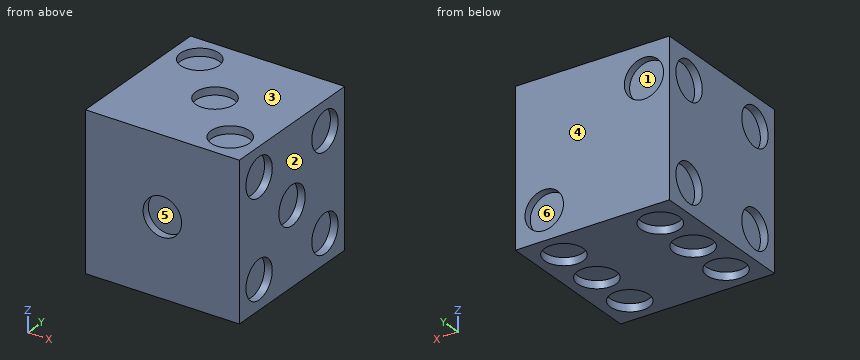
from build123d import *

# Parameters (mm, degrees)
F0_W      = 8
F0_H      = 8
F1_DEPTH  = 8
F2_R      = 1
F3_DEPTH  = 0.4
F4_R      = 1
F4_R_2    = 1.018966
F5_DEPTH  = 0.4
F6_R      = 1
F7_DEPTH  = 0.4
F8_R      = 1
F9_DEPTH  = 0.4
F10_R     = 1
F11_DEPTH = 0.4
F12_R     = 1
F13_DEPTH = 0.4


with BuildPart() as f1:
    # F0 (on Front) → F1 (new body)
    with BuildSketch(Plane.XZ):
        with Locations((2.040328, 4.226393)):
            Rectangle(F0_W, F0_H)
    extrude(amount=F1_DEPTH)

    # F2 (on face) → F3 (cut)
    with BuildSketch(Plane.XZ.offset(8)):
        with Locations((2.040328, 4.226393)):
            Circle(F2_R)
    extrude(amount=-F3_DEPTH, mode=Mode.SUBTRACT)

    # F4 (on face) → F5 (cut)
    with BuildSketch(Plane(origin=(0, 0, 0), x_dir=(-1, 0, 0), z_dir=(0, 1, 0))):
        with Locations((-4.540328, 1.726393)):
            Circle(F4_R)
        with Locations((0.640184, 6.564468)):
            Circle(F4_R_2)
    extrude(amount=-F5_DEPTH, mode=Mode.SUBTRACT)

    # F6 (on face) → F7 (cut)
    with BuildSketch(Plane(origin=(-1.959672, 0, 0), x_dir=(0, -1, 0), z_dir=(-1, 0, 0))):
        with Locations((6.5, 6.726393)):
            Circle(F6_R)
        with Locations((1.5, 6.726393)):
            Circle(F6_R)
        with Locations((1.5, 1.726393)):
            Circle(F6_R)
        with Locations((6.5, 1.726393)):
            Circle(F6_R)
    extrude(amount=-F7_DEPTH, mode=Mode.SUBTRACT)

    # F8 (on face) → F9 (cut)
    with BuildSketch(Plane.YZ.offset(6.040328)):
        with Locations((-4, 4.226393)):
            Circle(F8_R)
        with Locations((-6.5, 6.726393)):
            Circle(F8_R)
        with Locations((-1.5, 6.726393)):
            Circle(F8_R)
        with Locations((-1.5, 1.726393)):
            Circle(F8_R)
        with Locations((-6.5, 1.726393)):
            Circle(F8_R)
    extrude(amount=-F9_DEPTH, mode=Mode.SUBTRACT)

    # F10 (on face) → F11 (cut)
    with BuildSketch(Plane.XY.offset(8.226393)):
        with Locations((-0.459672, -1.5)):
            Circle(F10_R)
        with Locations((2.040328, -4)):
            Circle(F10_R)
        with Locations((4.540328, -6.5)):
            Circle(F10_R)
    extrude(amount=-F11_DEPTH, mode=Mode.SUBTRACT)

    # F12 (on face) → F13 (cut)
    with BuildSketch(Plane(origin=(0, 0, 0.226393), x_dir=(1, 0, 0), z_dir=(0, 0, -1))):
        with Locations((-0.459672, 6.5)):
            Circle(F12_R)
        with Locations((-0.459672, 4)):
            Circle(F12_R)
        with Locations((-0.459672, 1.5)):
            Circle(F12_R)
        with Locations((4.540328, 1.5)):
            Circle(F12_R)
        with Locations((4.540328, 4)):
            Circle(F12_R)
        with Locations((4.540328, 6.5)):
            Circle(F12_R)
    extrude(amount=-F13_DEPTH, mode=Mode.SUBTRACT)


solid = f1.part
Here's how the part is built. I have some questions about the finished solid (model axes, mm). Face numbers are marked on the shaded views. A direction names the side the tool comes from. Give positions to 0.01 mm unless a question says otherwise; leave off trailing zeros. Order: outer loops, then holes, each group sorted by start corner. A loop starts at its lowest first (then second) coordinate and runs counter-clockwise, first axis right, second up. Notation, with made-up numbers: (80, 85.25) -> (118, 85.25) arc R18 cw to (118, 98.25) -> close; hole circle Ø1 at (22, -36). An arc over 180 degrees is marked (long way). One line per item, written item: value. Start each with the question number.
1. Will these pins go through, and if not, where does the flat tip stop? pin 1 Ø1 at (y, z) = (-7, 6) entering from -X; pin 2 Ø1.6 at (y, z) = (-6.5, 6.73) entering from +X; pin 3 Ø0.6 at (x, z) = (2.5, 4) entering from -Y; pin 4 Ø0.6 at (x, y) = (4, -4) entering from -Z.
2. Imagine slicing it at B-B, the plane z = 1. List the corners of the cut face in (x, y) for me, plus the area to 3 significant figures.
3. Imagine slicing it at A-A, the plane y = -4. List the corners of the cut face in (x, z) for me.
4. For the marked faces 4, 5 and 6, which set-ups out of +Z, -Z, +X, -X, +Y, -Y let a thin tool reach every point of the face, with its end or its side?
5. I need wall thicknesses on probe 1 along X at (y, z) = (-1.5, 0.35); probe 2 along Z at (x, y) = (5.9, -6.5); probe 3 along Z at (x, y) = (4.25, -3.5). Which ranges of each line are inside material? Lowest first, please. Write a range as from..to.
6. Imagine slicing it at C-C, the plane x = 2. List the corners of the cut face in (y, z) for me, plus the area to 3 significant figures.
7. We'd pull the mould along X, two halves only. Please class the marked faces 1, 2 and 3: released by +X, released by -X, zero draft, split by the parting line, or undercut.
Values follow:
1. pin 1: stops at x = -1.96
1. pin 2: stops at x = 5.64
1. pin 3: stops at y = -7.6
1. pin 4: stops at z = 0.63
2. outline: (-1.96, -8) -> (6.04, -8) -> (6.04, -7.19) -> (5.64, -7.19) -> (5.64, -5.81) -> (6.04, -5.81) -> (6.04, -2.19) -> (5.64, -2.19) -> (5.64, -0.81) -> (6.04, -0.81) -> (6.04, 0) -> (5.23, 0) -> (5.23, -0.4) -> (3.85, -0.4) -> (3.85, 0) -> (-1.96, 0) -> (-1.96, -0.81) -> (-1.56, -0.81) -> (-1.56, -2.19) -> (-1.96, -2.19) -> (-1.96, -5.81) -> (-1.56, -5.81) -> (-1.56, -7.19) -> (-1.96, -7.19) -> close
2. area: 61.3 mm2
3. outline: (-1.96, 0.23) -> (-1.46, 0.23) -> (-1.46, 0.63) -> (0.54, 0.63) -> (0.54, 0.23) -> (3.54, 0.23) -> (3.54, 0.63) -> (5.54, 0.63) -> (5.54, 0.23) -> (6.04, 0.23) -> (6.04, 3.23) -> (5.64, 3.23) -> (5.64, 5.23) -> (6.04, 5.23) -> (6.04, 8.23) -> (3.04, 8.23) -> (3.04, 7.83) -> (1.04, 7.83) -> (1.04, 8.23) -> (-1.96, 8.23) -> close
4. face 4: +Z, -Z, +X, -X, +Y
4. face 5: -Y
4. face 6: +Y
5. probe 1: x = -1.96..-1.46, 0.54..3.54, 5.54..6.04
5. probe 2: z = 0.23..0.73, 2.73..5.73, 7.73..8.23
5. probe 3: z = 0.63..8.23
6. outline: (-8, 0.23) -> (0, 0.23) -> (0, 8.23) -> (-3, 8.23) -> (-3, 7.83) -> (-5, 7.83) -> (-5, 8.23) -> (-8, 8.23) -> (-8, 5.23) -> (-7.6, 5.23) -> (-7.6, 3.23) -> (-8, 3.23) -> close
6. area: 62.4 mm2
7. face 1: undercut
7. face 2: released by +X
7. face 3: zero draft
